```python
from build123d import *

# Parameters (mm, degrees)
SKETCH1_W           = 8.128
SKETCH1_H           = 16.51
BOSS_EXTRUDE1_DEPTH = 20.32
SKETCH2_R           = 2.493155922
BOSS_EXTRUDE2_DEPTH = 10.16
FILLET2_R           = 1.27
SKETCH3_W           = 8.89
SKETCH3_H           = 3.81
BOSS_EXTRUDE3_DEPTH = 3.556
FILLET3_R           = 1.27
BOSS_EXTRUDE4_DEPTH = 12.7
FILLET4_R           = 3.81


with BuildPart() as part:
    # Sketch1 → Boss-Extrude1 (new body)
    with BuildSketch(Plane(origin=(0, 0, 0), x_dir=(1, 0, 0), z_dir=(0, 1, 0))):
        Rectangle(SKETCH1_W, SKETCH1_H)
    extrude(amount=BOSS_EXTRUDE1_DEPTH)

    # Sketch2 → Boss-Extrude2 (add)
    with BuildSketch(Plane.ZY.offset(4.064)):
        with Locations(Location((4.445, 4.237080477, 0), (0, 0, 180))):
            Circle(SKETCH2_R)
    extrude(amount=BOSS_EXTRUDE2_DEPTH)

    # Fillet2
    fillet2_edges = [part.edges().sort_by_distance(p)[0] for p in [
        (-4.064, 4.237080477, 6.938155922),
    ]]
    fillet(fillet2_edges, radius=FILLET2_R)

    # Sketch3 → Boss-Extrude3 (add)
    with BuildSketch(Plane(origin=(4.064, 0, 0), x_dir=(0, 0, -1), z_dir=(1, 0, 0))):
        with Locations((0, 1.905)):
            Rectangle(SKETCH3_W, SKETCH3_H)
    extrude(amount=BOSS_EXTRUDE3_DEPTH)

    # Fillet3
    fillet3_edges = [part.edges().sort_by_distance(p)[0] for p in [
        (4.064, 3.81, 0),
    ]]
    fillet(fillet3_edges, radius=FILLET3_R)

    # Sketch5 → Boss-Extrude4 (add)
    with BuildSketch(Plane(origin=(0, 0, 0), x_dir=(-1, 0, 0), z_dir=(0, -1, 0))):
        Polygon((-10.16, -10.16), (-7.62, -10.16), (-7.62, 10.16), (-10.16, 10.16), (-18.612950502, 1.27), (-16.51, 1.27), (-10.16, 7.948319006), (-10.16, -7.948319006), (-16.51, -1.27), (-18.612950502, -1.27), align=None)
    extrude(amount=-BOSS_EXTRUDE4_DEPTH)

    # Fillet4
    # the kernel refuses this fillet: 3.81 mm, written as the material it adds along each edge
    with BuildSketch(Plane(origin=(7.62, 3.81, 4.445), x_dir=(0, 1, 0), z_dir=(0, 0, -1))) as fillet4_piece_1:
        with BuildLine():
            CenterArc((3.49192268, -3.81), FILLET4_R, 90, 66.421821522)
            Line((0, -2.286), (0, 0))
            Line((0, 0), (3.49192268, 0))
        make_face()
    extrude(amount=8.89)


solid = part.part
```
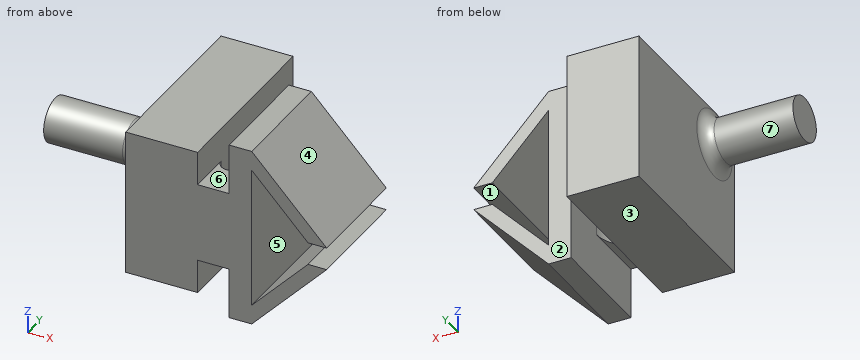
The listing builds one solid part. Answer for the finished solid, in the listing's coordinates (mm). Face numbers are marked on the shaded views. A direction names the side the tool comes from. Give positions to 0.01 mm unless a question says otherwise; leave off trailing zeros. Order: outer loops, then holes, each group sorted by start corner. A loop starts at its lowest first (then second) coordinate and runs counter-clockwise, first axis right, second up.
Item 1: The part is cut by section B-B, the plane x = 14. Give the vertices of the cut face in (y, z), and give its area (3 significant figures).
From the geometry:
outline: (0, -6.12) - (12.7, -6.12) - (12.7, -3.91) - (0, -3.91) - close; (0, 3.91) - (12.7, 3.91) - (12.7, 6.12) - (0, 6.12) - close
area: 56.2 mm2
Item 2: For a pull along X with two mould halves and no side action, classify the marked faces 4, 5, 6 and 7 as pulls with the +X half, pulls with the -X half, needs draft (parallel to the pull), parting line crosses it, or undercut.
From the geometry:
face 4: pulls with the +X half
face 5: undercut
face 6: undercut
face 7: needs draft
Item 3: The part is cut by section C-C, the plane z = -1.75. Give the vertices of the cut face in (x, y), and give its area (3 significant figures).
From the geometry:
outline: (-4.06, 0) - (10.16, 0) - (10.16, 12.7) - (7.62, 12.7) - (7.62, 7.3) arc R3.81 cw to (5.33, 3.81) arc R1.27 cw to (4.06, 5.08) - (4.06, 20.32) - (-4.06, 20.32) - close; (16.05, 0) - (18.16, 0) - (18.16, 12.7) - (16.05, 12.7) - close
area: 240 mm2
Item 4: Find the intervals of material crossed by probe 1 along X at (y, z) = (12.25, 1.75); probe 2 along X at (y, z) = (3, 6.5); probe 3 along Z at (x, y) = (7.5, 4.75) (3 decimals), in increasing order.
From the geometry:
probe 1: x = -4.06 to 4.06, 7.62 to 10.16, 16.05 to 18.16
probe 2: x = -14.22 to 4.06, 7.62 to 10.16, 11.54 to 13.64
probe 3: z = -4.445 to 4.445
Item 5: The part is cut by section D-D, the plane x = -1.5. Give the vertices of the cut face in (y, z) (3 decimals), and give its area (3 significant figures).
From the geometry:
outline: (0, -8.255) - (20.32, -8.255) - (20.32, 8.255) - (0, 8.255) - close
area: 335 mm2
Item 6: Which of the six approach directions +Z, -Z, +X, -X, +Y, -Y give full straight-line access (tool end or side, diameter ignored) to the marked faces 1, 2 and 3?
From the geometry:
face 1: +X, +Y, -Y
face 2: +Z, -Z, +X, +Y
face 3: -Z, -X, +Y, -Y
Item 7: Given pin 1 Ø8 at (y, z) = (8.5, 7) entering from +X; pin 2 Ø6.5 at (x, y) = (1.5, 7) entering from -Z (3 decimals); pin 3 Ø12 at (x, z) = (11, -0.5) entering from +Y, each flat-ended and moving along its own axis, determine where each tip first touches the part or whether it passes through.
From the geometry:
pin 1: stops at x = 16.97
pin 2: stops at z = -8.255
pin 3: stops at y = 12.7
Item 8: The part is cut by section A-A, the plane y = 10. Give the vertices of the cut face in (x, z) (3 decimals), and give its area (3 significant figures).
From the geometry:
outline: (-4.064, -8.255) - (4.064, -8.255) - (4.064, 8.255) - (-4.064, 8.255) - close; (7.62, -10.16) - (10.16, -10.16) - (18.613, -1.27) - (16.51, -1.27) - (10.16, -7.948) - (10.16, 7.948) - (16.51, 1.27) - (18.613, 1.27) - (10.16, 10.16) - (7.62, 10.16) - close
area: 219 mm2
